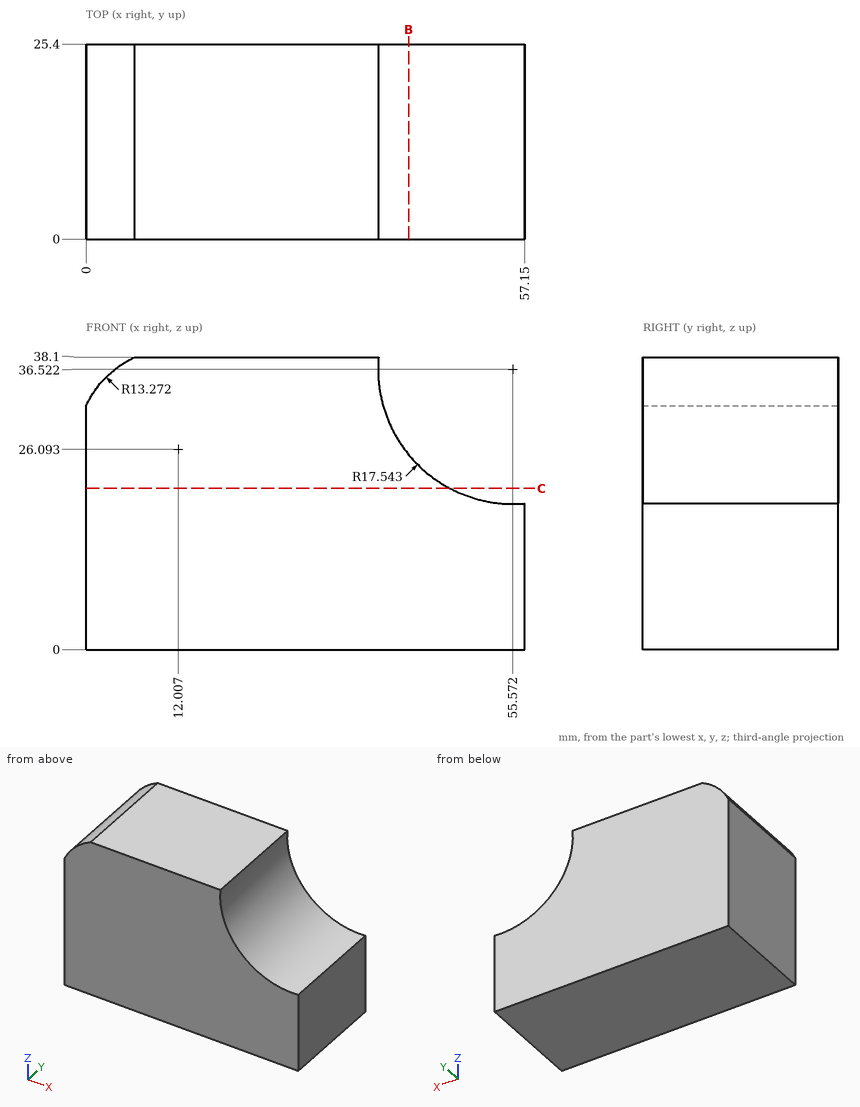
The drawing under review shows one solid part. Ordinate dimensions are in mm from its lowest x, y, z. Coordinates: 2 decimals unless noted, no trailing zeros. Loops run counter-clockwise (first coordinate to the right, second up) from the corner with the lowest first, then second, coordinate; pieces in that order, holes last. Notation, with made-up numbers: (54, 69) -> (102, 69) arc R24 ccw to (102, 94) -> close; hole circle Ø2 at (70, 30.5). An arc over 180 degrees is marked (long way). Answer as a JSON object with one key per item and string values.
Q1. Take a section at B-B on x = 42. Give the boundary of the cut face in (y, z).
Answer block:
{"outline": "(0, 0) -> (25.4, 0) -> (25.4, 25.41) -> (0, 25.41) -> close"}
Q2. Clearance check with a flat-ended pin moving along its axis: pin 1 Ø5 at (y, z) = (14.5, 27) entering from +X (1 decimal). State where the tip first meets the part, or that it passes through.
Answer block:
{"pin 1": "stops at x = 42.8"}
Q3. To check wall thickness, follow L1, parallel to X at y = 10.5, z = 21 (1 decimal); L2, parallel to X at y = 13.5, z = 34 (1 decimal); L3, parallel to Z at x = 41.5, y = 22.25 (1 decimal). State the ranges of each line that lie inside material, in increasing order.
Answer block:
{"L1": "x = 0 to 47.4", "L2": "x = 1.3 to 38.2", "L3": "z = 0 to 26"}
Q4. Take a section at C-C on z = 21. Give the boundary of the cut face in (x, y), plus the area to 3 significant figures.
Answer block:
{"outline": "(0, 0) -> (47.4, 0) -> (47.4, 25.4) -> (0, 25.4) -> close", "area": "1,200 mm^2"}
